Model file for the job. Use its own axes, mm. Face numbers are marked on the shaded views. A direction names the side the tool comes from. Give positions to 0.01 mm unless a question says otherwise; leave off trailing zeros. Loops run counter-clockwise (first coordinate to the right, second up) from the corner with the lowest first, then second, coordinate; pieces in that order, holes last. Notation, with made-up numbers: (21.25, -6) - (75.25, -6) arc R30 ccw to (75.25, 33) - close; hole circle Ø10 at (54, 3). An arc over 180 degrees is marked (long way). Use a Markdown table: item, result.
from build123d import *

# Parameters (mm, degrees)
SKETCH1_W               = 22.225
SKETCH1_H               = 43
BOSS_EXTRUDE1_DEPTH     = 6
SKETCH3_R               = 10
BOSS_EXTRUDE2_DEPTH     = 22.225
CUT_EXTRUDE1_DEPTH      = 28.47248908
CUT_EXTRUDE1_DEPTH_BACK = 28.47248908
SKETCH4_W               = 17
SKETCH4_H               = 37.5
CUT_EXTRUDE2_DEPTH      = 28.47248908
CUT_EXTRUDE2_DEPTH_BACK = 28.47248908
SKETCH5_R               = 3.175
BOSS_EXTRUDE3_DEPTH     = 6
M3_CLEARANCE_HOLE1_D    = 3.4
FILLET1_R               = 3
FILLET2_R               = 3
BOSS_EXTRUDE4_DEPTH     = 6


with BuildPart() as part:
    # Sketch1 → Boss-Extrude1 (new body)
    with BuildSketch(Plane(origin=(0, 0, 0), x_dir=(1, 0, 0), z_dir=(0, 1, 0))):
        Rectangle(SKETCH1_W, SKETCH1_H)
    extrude(amount=-BOSS_EXTRUDE1_DEPTH)

    # Sketch3 → Boss-Extrude2 (add)
    with BuildSketch(Plane(origin=(11.1125, 0, 0), x_dir=(0, 0, -1), z_dir=(1, 0, 0))):
        with Locations((0, -3)):
            Circle(SKETCH3_R)
    extrude(amount=-BOSS_EXTRUDE2_DEPTH)

    # Sketch4 → Cut-Extrude1 (cut, two sides: drawn at the far end of the back side and taken through both)
    with BuildSketch(Plane(origin=(0, 0, 0), x_dir=(1, 0, 0), z_dir=(0, 1, 0)).offset(-CUT_EXTRUDE1_DEPTH_BACK)):
        Rectangle(SKETCH4_W, SKETCH4_H)
    extrude(amount=CUT_EXTRUDE1_DEPTH + CUT_EXTRUDE1_DEPTH_BACK, mode=Mode.SUBTRACT)

    # Sketch5 → Cut-Extrude2 (cut, two sides: drawn at the far end of the back side and taken through both)
    with BuildSketch(Plane(origin=(0, 0, 0), x_dir=(0, 0, -1), z_dir=(1, 0, 0)).offset(-CUT_EXTRUDE2_DEPTH_BACK)):
        with Locations((0, -3)):
            Circle(SKETCH5_R)
    extrude(amount=CUT_EXTRUDE2_DEPTH + CUT_EXTRUDE2_DEPTH_BACK, mode=Mode.SUBTRACT)

    # Sketch7 → Boss-Extrude3 (add)
    with BuildSketch(Plane(origin=(0, 0, 0), x_dir=(1, 0, 0), z_dir=(0, 1, 0))):
        with BuildLine():
            Line((11.1125, 16.5), (13.1125, 16.5))
            ThreePointArc((13.1125, 16.5), (17.1125, 12.5), (13.1125, 8.5))
            Line((13.1125, 8.5), (11.1125, 8.5))
            Line((11.1125, 8.5), (11.1125, 16.5))
        make_face()
        with BuildLine():
            Line((11.1125, -16.5), (13.1125, -16.5))
            ThreePointArc((13.1125, -16.5), (17.1125, -12.5), (13.1125, -8.5))
            Line((13.1125, -8.5), (11.1125, -8.5))
            Line((11.1125, -8.5), (11.1125, -16.5))
        make_face()
        with BuildLine():
            Line((-11.1125, -8.5), (-11.1125, -16.5))
            Line((-11.1125, -16.5), (-13.1125, -16.5))
            ThreePointArc((-13.1125, -16.5), (-17.1125, -12.5), (-13.1125, -8.5))
            Line((-13.1125, -8.5), (-11.1125, -8.5))
        make_face()
        with BuildLine():
            Line((-11.1125, 8.5), (-11.1125, 16.5))
            Line((-11.1125, 16.5), (-13.1125, 16.5))
            ThreePointArc((-13.1125, 16.5), (-17.1125, 12.5), (-13.1125, 8.5))
            Line((-13.1125, 8.5), (-11.1125, 8.5))
        make_face()
    extrude(amount=-BOSS_EXTRUDE3_DEPTH)

    # M3 Clearance Hole1 (through all)
    with Locations(Plane(origin=(0, 0, 0), x_dir=(1, 0, 0), z_dir=(0, 1, 0))):
        with Locations((13.1125, 12.5), (-13.1125, 12.5), (-13.1125, -12.5), (13.1125, -12.5)):
            Hole(M3_CLEARANCE_HOLE1_D / 2)

    # Fillet1
    fillet1_edges = [part.edges().sort_by_distance(p)[0] for p in [
        (11.1125, -3, 21.5),
        (-11.1125, -3, 21.5),
        (-11.1125, -3, -21.5),
        (11.1125, -3, -21.5),
    ]]
    fillet(fillet1_edges, radius=FILLET1_R)

    # Fillet2
    fillet2_edges = [part.edges().sort_by_distance(p)[0] for p in [
        (-8.5, -3, -18.75),
        (8.5, -3, 18.75),
        (-8.5, -3, 18.75),
        (8.5, -3, -18.75),
    ]]
    fillet(fillet2_edges, radius=FILLET2_R)

    # Sketch11 → Boss-Extrude4 (add)
    with BuildSketch(Plane(origin=(0, 0, 0), x_dir=(1, 0, 0), z_dir=(0, 1, 0))):
        with BuildLine():
            Line((-15.5125, -9.3), (-11.1125, -6))
            Line((-11.1125, -6), (-11.1125, -8.5))
            Line((-11.1125, -8.5), (-13.1125, -8.5))
            ThreePointArc((-13.1125, -8.5), (-14.377411064, -8.705266808), (-15.5125, -9.3))
        make_face()
        with BuildLine():
            Line((-11.1125, 8.5), (-13.1125, 8.5))
            ThreePointArc((-13.1125, 8.5), (-14.377411064, 8.705266808), (-15.5125, 9.3))
            Line((-15.5125, 9.3), (-11.1125, 6))
            Line((-11.1125, 6), (-11.1125, 8.5))
        make_face()
        with BuildLine():
            Line((15.5125, 9.3), (11.1125, 6))
            Line((11.1125, 6), (11.1125, 8.5))
            Line((11.1125, 8.5), (13.1125, 8.5))
            ThreePointArc((13.1125, 8.5), (14.377411064, 8.705266808), (15.5125, 9.3))
        make_face()
        with BuildLine():
            Line((11.1125, -8.5), (13.1125, -8.5))
            ThreePointArc((13.1125, -8.5), (14.377411064, -8.705266808), (15.5125, -9.3))
            Line((15.5125, -9.3), (11.1125, -6))
            Line((11.1125, -6), (11.1125, -8.5))
        make_face()
    extrude(amount=-BOSS_EXTRUDE4_DEPTH)


solid = part.part
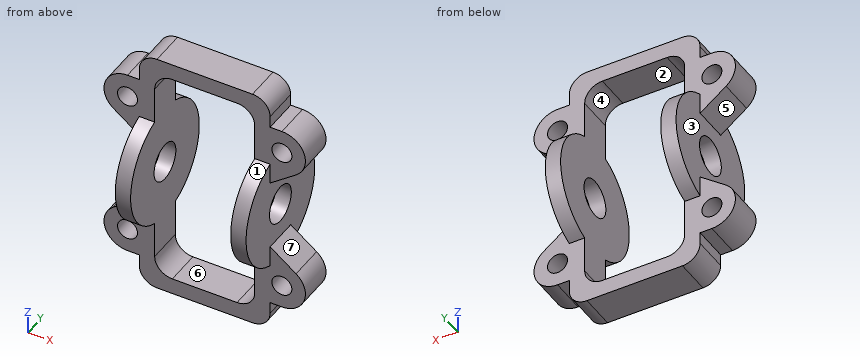
(1) Drill centre lines: probe 1 along X at (y, z) = (-4.4, 12.5); probe 2 along Z at (x, y) = (13, -3.75); probe 3 along Z at (x, y) = (1.5, -4). Where is each one in solid material? Low to high. Write a range as [from, to].
Computed:
| item | result |
|---|---|
| probe 1 | [-17.11, -14.81], [-11.41, -8.5], [8.5, 11.41], [14.81, 17.11] |
| probe 2 | [-16.5, -14.2], [-10.8, -7.42], [7.42, 10.8], [14.2, 16.5] |
| probe 3 | [-21.5, -18.75], [18.75, 21.5] |
(2) Mould opens along X. For the marked faces 4, 5, 6 and 7 say: pulls with the +X half, pulls with the -X half, needs draft (parallel to the pull), parting line crosses it, or undercut.
Computed:
| item | result |
|---|---|
| face 4 | undercut |
| face 5 | pulls with the -X half |
| face 6 | undercut |
| face 7 | pulls with the +X half |
(3) Slice it at C-C, the plane y = 4.25. Write the cut outline in (x, z), plus the area to 3 significant figures.
Computed:
| item | result |
|---|---|
| outline | (-11.11, -6.89) - (-8.5, -6.89) - (-8.5, 6.89) - (-11.11, 6.89) - close; (8.5, -6.89) - (11.11, -6.89) - (11.11, 6.89) - (8.5, 6.89) - close |
| area | 72.0 mm² |
(4) Slice it at B-B, the plane y = -3. Count the separate pieces of the cut face and the enclosed holes in it, plus the area to 3 significant figures.
Computed:
| item | result |
|---|---|
| separate pieces | 2 |
| enclosed holes | 4 |
| area | 431 mm² |
(5) Slice it at A-A, the plane z = 12.5. Write the cut outline in (x, y).
Computed:
| item | result |
|---|---|
| outline | (-17.11, -6) - (-14.81, -6) - (-14.81, 0) - (-17.11, 0) - close; (-11.41, -6) - (-8.5, -6) - (-8.5, 0) - (-11.41, 0) - close; (8.5, -6) - (11.41, -6) - (11.41, 0) - (8.5, 0) - close; (14.81, -6) - (17.11, -6) - (17.11, 0) - (14.81, 0) - close |
(6) Slice it at D-D, the plane z = 2. Write the cut outline in (x, y).
Computed:
| item | result |
|---|---|
| outline | (-11.11, -12.8) - (-8.5, -12.8) - (-8.5, -5.47) - (-11.11, -5.47) - close; (-11.11, -0.53) - (-8.5, -0.53) - (-8.5, 6.8) - (-11.11, 6.8) - close; (8.5, -12.8) - (11.11, -12.8) - (11.11, -5.47) - (8.5, -5.47) - close; (8.5, -0.53) - (11.11, -0.53) - (11.11, 6.8) - (8.5, 6.8) - close |
(7) Pin check, flat tips, straight feed: P1, Ø1.6, axis at x = 12, y = -2, coming from the +Z side; P2, Ø6, axis at x = 3, z = 16, coming from the +Y side; P3, Ø5, axis at y = -10, z = -2.5, coming from the +X side; P4, Ø2.5, axis at x = -13.11, z = 12.5, coming from the +Y side. Stop position of each tip, or through.
Computed:
| item | result |
|---|---|
| P1 | z = 16.5 |
| P2 | y = 0 |
| P3 | x = 11.11 |
| P4 | through |
(8) 3-axis set-ups, long thin cutter, end or side, ignore diameter. For the marked faces 1, 2 and 3: which of +Z, -Z, +X, -X, +Y, -Y reach the whole face in a straight line?
Computed:
| item | result |
|---|---|
| face 1 | +X, -X, -Y |
| face 2 | +Y, -Y |
| face 3 | -X |
